Could you check a few things on this model? Use its own coordinates, in mm. Face numbers are marked on the shaded views. A direction names the side the tool comes from. Coordinates: 2 decimals unless noted, no trailing zeros. Loops run counter-clockwise (first coordinate to the right, second up) from the corner with the lowest first, then second, coordinate; pieces in that order, holes last. Notation, with made-up numbers: (84, 13) - (127, 13) arc R15 cw to (127, 41) - close; hole circle Ø3 at (47.25, 5.5). An arc over 180 degrees is marked (long way). One line per item, written item: value. Start each with the question number.
(1) If we section it at A-A on y = 34: Write out the boundary of the cut face in (x, z).
(2) If I drill on line 1 along Y through (x, z) = (47, -30.5) (3 decimals); line 2 along Z through (x, y) = (19.5, 18.5); line 3 along Z through (x, y) = (21, 29.5), over which ranges is the centre line in solid material (lowest first)? Write a range as from..to.
(3) I'm going to push flat-ended pins straight in: P1, Ø1, axis at x = 41, y = 126, coming from the +Z side (3 decimals); P2, Ø1, axis at y = 38.5, z = -32, coming from the -X side (3 decimals). Where does each tip first touch, or does it pass through?
(4) If we section it at B-B on y = 60: Write out the boundary of the cut face in (x, z) (3 decimals), then the cut area to 3 significant figures.
(5) On a 3-axis mill with a long thin cutter (end or side, diameter ignored), from which of +Z, -Z, +X, -X, +Y, -Y can I reach the whole of each face in a straight line? I mean the marked faces 4, 5, 6, 7 and 8. Say none if no direction works.
(6) If we mould it in two halves opening along Y, with no side actions, what happens to the marked faces 1, 2 and 3? For each: pulls with the +Y half, pulls with the -Y half, needs draft (parallel to the pull), parting line crosses it, or undercut.
(7) If we section it at C-C on x = 35: Count the separate pieces of the cut face and the enclosed holes in it, then the cut area to 3 significant figures.
```python
from build123d import *

# Parameters (mm, degrees)
SKETCH1_W                    = 50.8
SKETCH1_H                    = 50.8
SKETCH1_W_2                  = 38.1
SKETCH1_H_2                  = 38.1
BOSS_EXTRUDE1_DEPTH          = 178
SKETCH2_W                    = 44.8
SKETCH2_H                    = 44.8
SKETCH2_W_2                  = 38.1
SKETCH2_H_2                  = 38.1
CUT_EXTRUDE1_DEPTH           = 20
SKETCH3_W                    = 46.8
SKETCH3_H                    = 124.475000116
CUT_EXTRUDE2_DEPTH           = 47.625
SKETCH4_W                    = 50.8
SKETCH4_H                    = 3.175
CUT_EXTRUDE3_DEPTH           = 3.175
SKETCH5_W                    = 3.175
SKETCH5_H                    = 3.175
CUT_EXTRUDE4_DEPTH           = 192.951243809
CUT_EXTRUDE5_DEPTH           = 1
SKETCH7_W                    = 46.8
SKETCH7_H                    = 3.175
CUT_EXTRUDE6_DEPTH           = 1
FILLET1_R                    = 1.5875
CUT_EXTRUDE7_DEPTH           = 2.34442
M1_2X0_25_TAPPED_HOLE1_D     = 0.95
M1_2X0_25_TAPPED_HOLE1_DEPTH = 2.9997
M1_2X0_25_TAPPED_HOLE1_TIP   = 0.285408794
BOSS_EXTRUDE2_REACH          = 193.689
CUT_EXTRUDE8_REACH           = 193.951
SKETCH15_W                   = 30
SKETCH15_H                   = 6.8
FILLET2_R                    = 1.5875
CUT_EXTRUDE9_DEPTH           = 21.8
CUT_EXTRUDE9_DEPTH_BACK      = 21.8
SKETCH20_R                   = 19.05


with BuildPart() as part:
    # Sketch1 → Boss-Extrude1 (new body)
    with BuildSketch(Plane(origin=(0, 0, 0), x_dir=(1, 0, 0), z_dir=(0, 1, 0))):
        with Locations((25.4, 25.4)):
            Rectangle(SKETCH1_W, SKETCH1_H)
        with Locations((25.4, 25.4)):
            Rectangle(SKETCH1_W_2, SKETCH1_H_2, mode=Mode.SUBTRACT)
    extrude(amount=BOSS_EXTRUDE1_DEPTH)

    # Sketch2 → Cut-Extrude1 (cut)
    with BuildSketch(Plane.XZ):
        with Locations((25.4, -25.4)):
            Rectangle(SKETCH2_W, SKETCH2_H)
        with Locations((25.4, -25.4)):
            Rectangle(SKETCH2_W_2, SKETCH2_H_2, mode=Mode.SUBTRACT)
    extrude(amount=-CUT_EXTRUDE1_DEPTH, mode=Mode.SUBTRACT)

    # Sketch3 → Cut-Extrude2 (cut)
    with BuildSketch(Plane.XY):
        with Locations((25.4, 109.412499942)):
            Rectangle(SKETCH3_W, SKETCH3_H)
    extrude(amount=-CUT_EXTRUDE2_DEPTH, mode=Mode.SUBTRACT)

    # Sketch4 → Cut-Extrude3 (cut)
    with BuildSketch(Plane.XY):
        with Locations((25.4, 25.5875)):
            Rectangle(SKETCH4_W, SKETCH4_H)
        with Locations((25.4, 38.5875)):
            Rectangle(SKETCH4_W, SKETCH4_H)
    cut_extrude3 = extrude(amount=-CUT_EXTRUDE3_DEPTH, mode=Mode.SUBTRACT)

    # Sketch5 → Cut-Extrude4 (cut, through all)
    with BuildSketch(Plane.XY):
        with Locations((1.5875, 38.5875)):
            Rectangle(SKETCH5_W, SKETCH5_H)
        with Locations((1.5875, 25.5875)):
            Rectangle(SKETCH5_W, SKETCH5_H)
    cut_extrude4 = extrude(amount=-CUT_EXTRUDE4_DEPTH, mode=Mode.SUBTRACT)

    # Sketch6 → Cut-Extrude5 (cut)
    with BuildSketch(Plane.ZY):
        with BuildLine():
            Line((-32.4, 175), (-18.4, 175))
            ThreePointArc((-18.4, 175), (-17.4, 174), (-18.4, 173))
            Line((-18.4, 173), (-32.4, 173))
            ThreePointArc((-32.4, 173), (-33.4, 174), (-32.4, 175))
        make_face()
        with BuildLine():
            Line((-32.4, 171.5), (-18.4, 171.5))
            ThreePointArc((-18.4, 171.5), (-17.4, 170.5), (-18.4, 169.5))
            Line((-18.4, 169.5), (-32.4, 169.5))
            ThreePointArc((-32.4, 169.5), (-33.4, 170.5), (-32.4, 171.5))
        make_face()
        with BuildLine():
            Line((-32.4, 168), (-18.4, 168))
            ThreePointArc((-18.4, 168), (-17.4, 167), (-18.4, 166))
            Line((-18.4, 166), (-32.4, 166))
            ThreePointArc((-32.4, 166), (-33.4, 167), (-32.4, 168))
        make_face()
    cut_extrude5 = extrude(amount=-CUT_EXTRUDE5_DEPTH, mode=Mode.SUBTRACT)

    # Mirror1: Cut-Extrude3 across plane
    add(cut_extrude3.mirror(Plane.XY.offset(-25.4)), mode=Mode.SUBTRACT)

    # Mirror2: Cut-Extrude4, Cut-Extrude5 across plane
    add(cut_extrude4.mirror(Plane.ZY.offset(-25.4)), mode=Mode.SUBTRACT)
    add(cut_extrude5.mirror(Plane.ZY.offset(-25.4)), mode=Mode.SUBTRACT)

    # Sketch7 → Cut-Extrude6 (cut)
    with BuildSketch(Plane.XY):
        with Locations((25.4, 173.2375)):
            Rectangle(SKETCH7_W, SKETCH7_H)
        with Locations((25.4, 45.587499884)):
            Rectangle(SKETCH7_W, SKETCH7_H)
    extrude(amount=-CUT_EXTRUDE6_DEPTH, mode=Mode.SUBTRACT)

    # Fillet1
    fillet1_edges = [part.edges().sort_by_distance(p)[0] for p in [
        (47.8, 10, -3),
        (47.8, 10, -47.8),
        (2, 174.825, -0.5),
        (48.8, 174.825, -0.5),
        (3, 10, -47.8),
        (2, 43.999999884, -0.5),
        (3, 10, -3),
        (48.8, 43.999999884, -0.5),
        (2, 47.174999884, -24.3125),
        (2, 171.65, -24.3125),
        (48.8, 171.65, -24.3125),
        (48.8, 47.174999884, -24.3125),
    ]]
    fillet(fillet1_edges, radius=FILLET1_R)

    # Sketch8 → Cut-Extrude7 (cut)
    with BuildSketch(Plane(origin=(0, 178, 0), x_dir=(1, 0, 0), z_dir=(0, 1, 0))):
        with BuildLine():
            Line((4.7625, 49.2125), (46.0375, 49.2125))
            ThreePointArc((46.0375, 49.2125), (48.28256403, 48.28256403), (49.2125, 46.0375))
            Line((49.2125, 46.0375), (49.2125, 4.7625))
            ThreePointArc((49.2125, 4.7625), (48.28256403, 2.51743597), (46.0375, 1.5875))
            Line((46.0375, 1.5875), (4.7625, 1.5875))
            ThreePointArc((4.7625, 1.5875), (2.51743597, 2.51743597), (1.5875, 4.7625))
            Line((1.5875, 4.7625), (1.5875, 46.0375))
            ThreePointArc((1.5875, 46.0375), (2.51743597, 48.28256403), (4.7625, 49.2125))
        make_face()
    extrude(amount=-CUT_EXTRUDE7_DEPTH, mode=Mode.SUBTRACT)

    # M1.2x0.25 Tapped Hole1
    with Locations(Plane.XY.offset(-1)):
        with Locations((3.8415, 172.98375321), (46.95875321, 172.98375321), (3.8415, 45.841499884), (46.95875321, 45.841499884)):
            Hole(M1_2X0_25_TAPPED_HOLE1_D / 2, depth=M1_2X0_25_TAPPED_HOLE1_DEPTH)
            with Locations((0, 0, -(M1_2X0_25_TAPPED_HOLE1_DEPTH + M1_2X0_25_TAPPED_HOLE1_TIP / 2))):  # 118° drill point
                Cone(0, M1_2X0_25_TAPPED_HOLE1_D / 2, M1_2X0_25_TAPPED_HOLE1_TIP, mode=Mode.SUBTRACT)

    # Sketch17 → Boss-Extrude2 (add, up to next)
    with BuildSketch(Plane.XY.offset(-1), mode=Mode.PRIVATE) as boss_extrude2_sk1:
        with BuildLine():
            Line((2, 170.0625), (2, 48.762499884))
            ThreePointArc((2, 48.762499884), (2.464967985, 47.639967869), (3.5875, 47.174999884))
            Line((3.5875, 47.174999884), (5.5875, 47.174999884))
            ThreePointArc((5.5875, 47.174999884), (4.464967985, 47.639967869), (4, 48.762499884))
            Line((4, 48.762499884), (4, 170.0625))
            ThreePointArc((4, 170.0625), (4.464967985, 171.185032015), (5.5875, 171.65))
            Line((5.5875, 171.65), (3.5875, 171.65))
            ThreePointArc((3.5875, 171.65), (2.464967985, 171.185032015), (2, 170.0625))
        make_face()
    boss_extrude2_tool1 = extrude(boss_extrude2_sk1.sketch, amount=-BOSS_EXTRUDE2_REACH, mode=Mode.PRIVATE) - part.part
    add(boss_extrude2_tool1.solids().sort_by_distance((3.00869, 109.4125, -1))[0])

    # Sketch15 → Cut-Extrude8 (cut, up to next)
    with BuildSketch(Plane.ZY, mode=Mode.PRIVATE) as cut_extrude8_sk1:
        with Locations((-25.4, 105)):
            Rectangle(SKETCH15_W, SKETCH15_H)
    cut_extrude8_tool1 = extrude(cut_extrude8_sk1.sketch, amount=-CUT_EXTRUDE8_REACH, mode=Mode.PRIVATE) & part.part
    # Sketch15 → Cut-Extrude8 (cut, up to next)
    with BuildSketch(Plane.ZY, mode=Mode.PRIVATE) as cut_extrude8_sk2:
        with Locations((-25.4, 121.8)):
            Rectangle(SKETCH15_W, SKETCH15_H)
    cut_extrude8_tool2 = extrude(cut_extrude8_sk2.sketch, amount=-CUT_EXTRUDE8_REACH, mode=Mode.PRIVATE) & part.part
    add(cut_extrude8_tool1.solids().sort_by_distance((0, 105, -25.4))[0], mode=Mode.SUBTRACT)
    add(cut_extrude8_tool2.solids().sort_by_distance((0, 121.8, -25.4))[0], mode=Mode.SUBTRACT)

    # Fillet2
    fillet2_edges = [part.edges().sort_by_distance(p)[0] for p in [
        (2, 101.6, -10.4),
        (2, 108.4, -10.4),
        (2, 108.4, -40.4),
        (2, 101.6, -40.4),
        (2, 118.4, -10.4),
        (2, 125.2, -10.4),
        (2, 125.2, -40.4),
        (2, 118.4, -40.4),
    ]]
    fillet(fillet2_edges, radius=FILLET2_R)

    # Sketch20 → Cut-Extrude9 (cut, two sides: drawn at the far end of the back side and taken through both)
    with BuildSketch(Plane(origin=(0, 113.4, 0), x_dir=(1, 0, 0), z_dir=(0, 1, 0)).offset(-CUT_EXTRUDE9_DEPTH_BACK)):
        with Locations((-16.55, 25.4)):
            Circle(SKETCH20_R)
    extrude(amount=CUT_EXTRUDE9_DEPTH + CUT_EXTRUDE9_DEPTH_BACK, mode=Mode.SUBTRACT)


solid = part.part
```
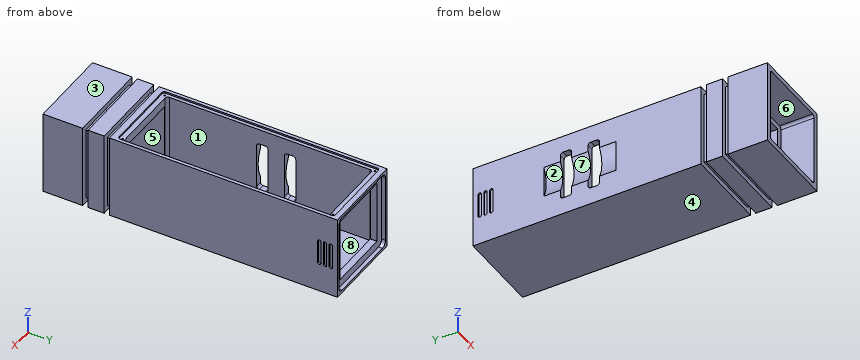
Values:
1. outline: (0, -50.8) - (50.8, -50.8) - (50.8, 0) - (0, 0) - close; hole (6.35, -44.45) - (44.45, -44.45) - (44.45, -6.35) - (6.35, -6.35) - close
2. line 1: y = 20..47.175, 171.65..175.656
2. line 2: z = -50.8..-47.8, -3..0
2. line 3: z = -50.8..-44.45, -6.35..0
3. P1: stops at z = -47.625
3. P2: stops at x = 3.175
4. outline: (0, -50.8) - (50.8, -50.8) - (50.8, 0) - (48.8, 0) - (48.8, -47.625) - (4, -47.625) - (4, -1) - (2, -1) - (2, 0) - (0, 0) - close
4. area: 445 mm2
5. face 4: -Z, +X, -X, +Y, -Y
5. face 5: +Y, -Y
5. face 6: -Y
5. face 7: -X
5. face 8: +Z
6. face 1: undercut
6. face 2: undercut
6. face 3: needs draft
7. separate pieces: 3
7. enclosed holes: 0
7. area: 872 mm2
